Part model, mm, in its own coordinate system. A direction names the side the tool comes from. Round coordinates to 2 decimals unless told otherwise and drop trailing zeros. Loops run counter-clockwise (first coordinate to the right, second up) from the corner with the lowest first, then second, coordinate; pieces in that order, holes last. Notation, with made-up numbers: M 79.5,-35.75 L 85.5,-35.75 A6 ccw 85.5,-29.75 Z; hole C -6.75,37.25 d3. An arc over 180 degrees is marked long. Put each result on its own line as item: value. Start each with the question number.
1) Probe line 1 along Y through (x, z) = (0, 0.2); line 2 along X through (y, z) = (0, 1.25); line 3 along X through (y, z) = (-10, 1.8). List the from-to ranges inside material, lowest first.
2) Which spindle directions (+Z, -Z, +X, -X, +Y, -Y) get a long thin tool onto all of the face, cutting with end or side? Do faces 1 (the flat face through (-0.85, -13.96, 1.29)), 2 (the cylindrical face through (-1.8, 12.57, 1.25)), 3 (the flat face through (-13.02, 5, 1.29)), 4 (the cylindrical face through (-10.68, 6.87, 1.25)). Say none if no direction does.
3) Slice it at B-B on x = 0. Give the cut face in (y, z), then the cut area to 3 significant figures.
4) Slice it at D-D on y = -8.5. Give the cut face in (x, z).
5) Pull direction Y, two halves, no side cores. Call faces 5 (the cylindrical face through (-0.496, -3.778, 0.161)), 6 (the flat face through (13.86, 6.34, 1.29)), 7 (the cylindrical face through (1.8, -12.57, 1.25)): +Y half, -Y half, draft (parallel to the pull), parting line (faces both ways), or undercut.
6) Drop flat-ended pins along their axis: pin 1 Ø2 at (x, y) = (-5, -8.5) entering from -Z; pin 2 Ø1.5 at (x, y) = (-6, 10.5) entering from -Z; pin 3 Ø6 at (x, y) = (0, 0) entering from -Z; pin 4 Ø2 at (y, z) = (11.5, 0) entering from +X. Give the stop position or say it passes through.
7) Slice it at C-C on z = -0.9. Give the cut face in (x, y).
8) Slice it at A-A on y = 0. Give the cut face in (x, z).
```python
from build123d import *

# Parameters (mm, degrees)
SKETCH3_R            = 12.7
BOSS_EXTRUDE2_DEPTH  = 2.54
BOSS_EXTRUDE4_DEPTH  = 2.54
CIRPATTERN1_COUNT    = 22
SKETCH5_R            = 11.43
BOSS_EXTRUDE6_DEPTH  = 0.254
SKETCH6_R            = 3.81
CUT_EXTRUDE1_DEPTH   = 16.08
SKETCH8_R            = 11.43
CUT_EXTRUDE2_DEPTH   = 0.254
SKETCH9_R            = 5.08
BOSS_EXTRUDE11_DEPTH = 2.54
CUT_EXTRUDE3_START   = -2.54
SKETCH10_R           = 3.81
CUT_EXTRUDE3_DEPTH   = 2.54


with BuildPart() as part:
    # Sketch3 → Boss-Extrude2 (new body)
    with BuildSketch(Plane.XY):
        Circle(SKETCH3_R)
    boss_extrude2 = extrude(amount=BOSS_EXTRUDE2_DEPTH)

    # Sketch4 → Boss-Extrude4 (add)
    with BuildSketch(Plane.XY.offset(2.54)):
        Polygon((-0.508, 15.24), (0.508, 15.24), (1.657370651, 10.950490333), (-1.657370651, 10.950490333), align=None)
    boss_extrude4 = extrude(amount=-BOSS_EXTRUDE4_DEPTH)

    # CirPattern1: Boss-Extrude2, Boss-Extrude4 ×22 about axis
    cirpattern1_axis = Axis((0, 0, 0), (0, 0, 1))
    add([boss_extrude2.rotate(cirpattern1_axis, i * 360 / CIRPATTERN1_COUNT) for i in range(1, CIRPATTERN1_COUNT)])
    add([boss_extrude4.rotate(cirpattern1_axis, i * 360 / CIRPATTERN1_COUNT) for i in range(1, CIRPATTERN1_COUNT)])

    # Sketch5 → Boss-Extrude6 (add)
    with BuildSketch(Plane(origin=(0, 0, 0), x_dir=(-1, 0, 0), z_dir=(0, 0, -1))):
        Circle(SKETCH5_R)
    extrude(amount=-BOSS_EXTRUDE6_DEPTH)

    # Sketch6 → Cut-Extrude1 (cut)
    with BuildSketch(Plane.XY.offset(2.54)):
        Circle(SKETCH6_R)
    extrude(amount=-CUT_EXTRUDE1_DEPTH, mode=Mode.SUBTRACT)

    # Sketch8 → Cut-Extrude2 (cut)
    with BuildSketch(Plane(origin=(0, 0, 0), x_dir=(-1, 0, 0), z_dir=(0, 0, -1))):
        Circle(SKETCH8_R)
    extrude(amount=-CUT_EXTRUDE2_DEPTH, mode=Mode.SUBTRACT)

    # Sketch9 → Boss-Extrude11 (add)
    with BuildSketch(Plane(origin=(0, 0, 0.254), x_dir=(-1, 0, 0), z_dir=(0, 0, -1))):
        Circle(SKETCH9_R)
    extrude(amount=BOSS_EXTRUDE11_DEPTH)

    # Sketch10 → Cut-Extrude3 (cut)
    with BuildSketch(Plane(origin=(0, 0, -2.286), x_dir=(-1, 0, 0), z_dir=(0, 0, -1)).offset(CUT_EXTRUDE3_START)):
        with Locations(Location((0, 0, 0), (0, 0, 180))):
            Circle(SKETCH10_R)
    extrude(amount=CUT_EXTRUDE3_DEPTH, mode=Mode.SUBTRACT)


solid = part.part
```
Recorded:
1. line 1: y = -15.24 to -11.43, -5.08 to -3.81, 3.81 to 5.08, 11.43 to 15.24
1. line 2: x = -12.7 to -3.81, 3.81 to 12.7
1. line 3: x = -11.5 to -10.44, -7.85 to 7.85, 10.44 to 11.5
2. face 1: +Z, -Z, -Y
2. face 2: +Z, -Z, +Y
2. face 3: +Z, -Z, -X
2. face 4: +Z, -Z
3. outline: M -15.24,0 L -11.43,0 L -11.43,0.25 L -5.08,0.25 L -5.08,-2.29 L -3.81,-2.29 L -3.81,2.54 L -15.24,2.54 Z; M 3.81,-2.29 L 5.08,-2.29 L 5.08,0.25 L 11.43,0.25 L 11.43,0 L 15.24,0 L 15.24,2.54 L 3.81,2.54 Z
3. area: 60.6 mm2
4. outline: M -11.11,0 L -7.64,0 L -7.64,0.25 L 7.64,0.25 L 7.64,0 L 11.11,0 L 11.11,2.54 L -11.11,2.54 Z
5. face 5: undercut
5. face 6: +Y half
5. face 7: -Y half
6. pin 1: stops at z = 0.25
6. pin 2: stops at z = 0
6. pin 3: passes through
6. pin 4: stops at x = 8.65
7. outline: C 0,0 d10.16; hole C 0,0 d7.62
8. outline: M -12.7,0 L -11.43,0 L -11.43,0.25 L -5.08,0.25 L -5.08,-2.29 L -3.81,-2.29 L -3.81,2.54 L -12.7,2.54 Z; M 3.81,-2.29 L 5.08,-2.29 L 5.08,0.25 L 11.43,0.25 L 11.43,0 L 12.7,0 L 12.7,2.54 L 3.81,2.54 Z
